Can you work these out from the model? Positions are in its coordinate system, mm. A direction names the side the tool comes from. Round coordinates to 2 decimals unless told otherwise and drop trailing zeros. Loops run counter-clockwise (first coordinate to the right, second up) from the corner with the lowest first, then second, coordinate; pieces in that order, holes last.
from build123d import *

# Parameters (mm, degrees)
SKETCH1_W              = 135
SKETCH1_H              = 135
BOSS_EXTRUDE1_DEPTH    = 40
SKETCH2_R              = 10
CUT_EXTRUDE1_DEPTH     = 104.501207722
SKETCH4_R              = 50
BOSS_EXTRUDE2_DEPTH    = 20
SKETCH5_R              = 45
BOSS_EXTRUDE3_DEPTH    = 5
SKETCH6_R              = 50
BOSS_EXTRUDE4_DEPTH    = 5
CHAMFER1_SIZE          = 2
SKETCH7_R              = 35
CUT_EXTRUDE2_DEPTH     = 65
M20X2_5_TAPPED_HOLE1_D = 17.5


with BuildPart() as part:
    # Sketch1 → Boss-Extrude1 (new body)
    with BuildSketch(Plane.XY):
        Rectangle(SKETCH1_W, SKETCH1_H)
    extrude(amount=BOSS_EXTRUDE1_DEPTH)

    # Sketch2 → Cut-Extrude1 (cut, through all)
    with BuildSketch(Plane.XY.offset(40)):
        with Locations((-47.5, 47.5)):
            Circle(SKETCH2_R)
        with Locations(Location((47.5, 47.5, 0), (0, 0, 180))):
            Circle(SKETCH2_R)
        with Locations((47.5, -47.5)):
            Circle(SKETCH2_R)
        with Locations(Location((-47.5, -47.5, 0), (0, 0, 180))):
            Circle(SKETCH2_R)
    extrude(amount=-CUT_EXTRUDE1_DEPTH, mode=Mode.SUBTRACT)

    # Sketch4 → Boss-Extrude2 (add)
    with BuildSketch(Plane.XY.offset(40)):
        Circle(SKETCH4_R)
    extrude(amount=BOSS_EXTRUDE2_DEPTH)

    # Sketch5 → Boss-Extrude3 (add)
    with BuildSketch(Plane.XY.offset(60)):
        Circle(SKETCH5_R)
    extrude(amount=BOSS_EXTRUDE3_DEPTH)

    # Sketch6 → Boss-Extrude4 (add)
    with BuildSketch(Plane.XY.offset(65)):
        Circle(SKETCH6_R)
    extrude(amount=BOSS_EXTRUDE4_DEPTH)

    # Chamfer1
    chamfer1_edges = [part.edges().sort_by_distance(p)[0] for p in [
        (-50, 0, 70),
    ]]
    chamfer(chamfer1_edges, length=CHAMFER1_SIZE)

    # Sketch7 → Cut-Extrude2 (cut)
    with BuildSketch(Plane.XY.offset(70)):
        Circle(SKETCH7_R)
    extrude(amount=-CUT_EXTRUDE2_DEPTH, mode=Mode.SUBTRACT)

    # M20x2.5 Tapped Hole1 (through all)
    with Locations(Plane(origin=(0, -67.5, 20), x_dir=(-1, 0, 0), z_dir=(0, -1, 0))):
        with Locations((0, 0)):
            Hole(M20X2_5_TAPPED_HOLE1_D / 2)


solid = part.part
(1) If we section it at D-D, the plane z = 45: List the corners of the cut face in (x, y) for me, then the cut area to 3 significant figures.
Worked answers:
outline: circle Ø100 at (0, 0); hole circle Ø70 at (0, 0)
area: 4,010 mm2
(2) If I drill on line 1 (Y direction, x = 0, z = 53); line 2 (Y direction, x = 47.5, z = 8); line 3 (Y direction, x = 55.5, z = 36.5), over which ranges is the centre line in solid material (lowest first)?
Worked answers:
line 1: y = -50 to -35, 35 to 50
line 2: y = -67.5 to -57.5, -37.5 to 37.5, 57.5 to 67.5
line 3: y = -67.5 to -53.5, -41.5 to 41.5, 53.5 to 67.5
(3) For faces 1 (the flat face through (-41, 19, 60)), 2 (the cylindrical face through (32.33, -13.41, 37.96)), 3 (the flat face through (-1, -67.5, 11)), which set-ups out of +Z, -Z, +X, -X, +Y, -Y let a thin tool reach every point of the face, with its end or its side?
Worked answers:
face 1: none
face 2: +Z
face 3: +Z, -Z, +X, -X, -Y
(4) If we section it at A-A, the plane z = 20: List the corners of the cut face in (x, y) for me.
Worked answers:
outline: (-67.5, -67.5) - (-8.75, -67.5) - (-8.75, -33.89) arc R35 cw to (-8.75, 33.89) - (-8.75, 67.5) - (-67.5, 67.5) - close; (8.75, -67.5) - (67.5, -67.5) - (67.5, 67.5) - (8.75, 67.5) - (8.75, 33.89) arc R35 cw to (8.75, -33.89) - close; hole circle Ø20 at (-47.5, -47.5); hole circle Ø20 at (-47.5, 47.5); hole circle Ø20 at (47.5, -47.5); hole circle Ø20 at (47.5, 47.5)
(5) Will these pins go through, and if not, where does the flat tip stop? P1, Ø3, axis at x = 12.5, z = 48, coming from the +Y side (3 decimals); P2, Ø10, axis at x = -10.5, z = 51.5, coming from the +Y side.
Worked answers:
P1: stops at y = 48.775
P2: stops at y = 49.7
(6) If we section it at B-B, the plane z = 34: List the corners of the cut face in (x, y) for me.
Worked answers:
outline: (-67.5, -67.5) - (67.5, -67.5) - (67.5, 67.5) - (-67.5, 67.5) - close; hole circle Ø20 at (-47.5, -47.5); hole circle Ø20 at (-47.5, 47.5); hole circle Ø70 at (0, 0); hole circle Ø20 at (47.5, -47.5); hole circle Ø20 at (47.5, 47.5)
(7) If we section it at C-C, the plane y = -40.5: State how many separate pieces and enclosed holes the cut face has, then the cut area to 3 significant figures.
Worked answers:
separate pieces: 3
enclosed holes: 1
area: 5,670 mm2
(8) If we mould it in two halves opening along Z, with no side actions, what happens to faces 4 (the cylindrical face through (-1.139, 50.93, 11.324)), 5 (the flat face through (29, 46, 40)), 6 (the flat face through (-1, 1, 0))? For each: released by +Z, released by -Z, zero draft, split by the parting line, or undercut.
Worked answers:
face 4: undercut
face 5: released by +Z
face 6: released by -Z
